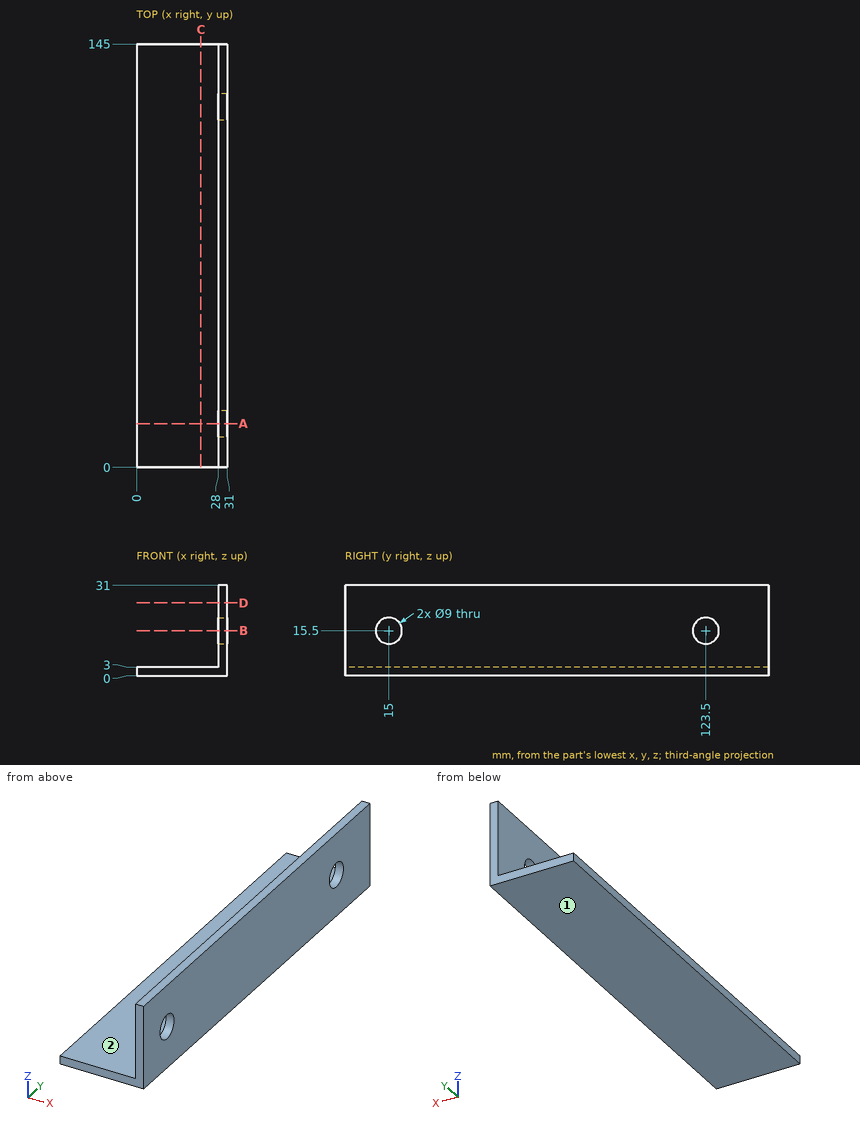
The figure shows three views and two pictorial views of one solid part (mm, origin at its lowest corner). Answer the questions. A direction names the side the tool comes from. Round coordinates to 2 decimals unless told otherwise and drop trailing zeros. Order: outer loops, then holes, each group sorted by start corner. A loop starts at its lowest first (then second) coordinate and runs counter-clockwise, first axis right, second up. Notation, with made-up numbers: (-35.5, -9.5) -> (-8.5, -9.5) arc R21 ccw to (-8.5, 2.5) -> close; hole circle Ø4 at (-12, 18.5). An arc over 180 degrees is marked (long way). One line per item, written item: value.
Item 1: Find section A-A, the plane y = 15. Give the vertices of the cut face in (x, z).
Taken from the geometry:
outline: (0, 0) -> (31, 0) -> (31, 11) -> (28, 11) -> (28, 3) -> (0, 3) -> close; (28, 20) -> (31, 20) -> (31, 31) -> (28, 31) -> close
Item 2: Straight lines are drawn through the part: L1, parallel to Y at x = 30, z = 15; L2, parallel to Z at x = 29, y = 123; L3, parallel to X at y = 28.5, z = 16. For each, find the intervals that lie inside material, in ascending order.
Taken from the geometry:
L1: y = 0 to 10.53, 19.47 to 119.03, 127.97 to 145
L2: z = 0 to 11.03, 19.97 to 31
L3: x = 28 to 31
Item 3: Find section D-D, the plane z = 25. Give the vertices of the cut face in (x, y), then the cut area to 3 significant figures.
Taken from the geometry:
outline: (28, 0) -> (31, 0) -> (31, 145) -> (28, 145) -> close
area: 435 mm2
Item 4: Given P1, Ø2, axis at x = 4.5, y = 64.5, coming from the +Z side; P2, Ø10, axis at y = 109.5, z = 24, coming from the -X side, each flat-ended and moving along its own axis, determine where each tip first touches the part or whether it passes through.
Taken from the geometry:
P1: stops at z = 3
P2: stops at x = 28
Item 5: Find section B-B, the plane z = 15.5. Give the vertices of the cut face in (x, y), then the cut area to 3 significant figures.
Taken from the geometry:
outline: (28, 0) -> (31, 0) -> (31, 10.5) -> (28, 10.5) -> close; (28, 19.5) -> (31, 19.5) -> (31, 119) -> (28, 119) -> close; (28, 128) -> (31, 128) -> (31, 145) -> (28, 145) -> close
area: 381 mm2
Item 6: For the marked faces 1 and 2, determine the directions among +Z, -Z, +X, -X, +Y, -Y from which every point of the face is accessible in a straight line to the end or side of a thin tool.
Taken from the geometry:
face 1: -Z, +X, -X, +Y, -Y
face 2: +Z, -X, +Y, -Y
Item 7: Find section C-C, the plane x = 22. Give the vertices of the cut face in (y, z).
Taken from the geometry:
outline: (0, 0) -> (145, 0) -> (145, 3) -> (0, 3) -> close
